from build123d import *

# Parameters (mm, degrees)
SKETCH1_R           = 1.7
BOSS_EXTRUDE1_DEPTH = 6.35
CHAMFER1_SIZE       = 1.7
SKETCH2_R           = 1.65
CUT_EXTRUDE1_DEPTH  = 10
FILLET1_R           = 3


with BuildPart() as part:
    # Sketch1 → Boss-Extrude1 (new body)
    with BuildSketch(Plane(origin=(7.6e-08, 0, -21.644897171), x_dir=(1, 0, 4e-09), z_dir=(-4e-09, 0, 1))):
        with BuildLine():
            Line((3.000021754, 7.262533291), (3.000021754, 1.9987))
            Line((3.000021754, 1.9987), (19.00000025, 1.9987))
            Line((19.00000025, 1.9987), (19.00000025, 22.8687))
            Line((19.00000025, 22.8687), (-19.00000025, 22.8687))
            Line((-19.00000025, 22.8687), (-19.00000025, 1.9987))
            Line((-19.00000025, 1.9987), (-3.409734271, 1.9987))
            Line((-3.409734271, 1.9987), (-3.409734271, 7.262533291))
            ThreePointArc((-3.409734271, 7.262533291), (-0.204856259, 10.467411304), (3.000021754, 7.262533291))
        make_face()
        with Locations((9.295143741, 7.262533291)):
            Circle(SKETCH1_R, mode=Mode.SUBTRACT)
        with Locations((-9.704856259, 7.262533291)):
            Circle(SKETCH1_R, mode=Mode.SUBTRACT)
    extrude(amount=BOSS_EXTRUDE1_DEPTH)

    # Chamfer1
    chamfer1_edges = [part.edges().sort_by_distance(p)[0] for p in [
        (7.595143795, 7.262533291, -15.294897144),
        (-11.404856205, 7.262533291, -15.294897211),
    ]]
    chamfer(chamfer1_edges, length=CHAMFER1_SIZE)

    # Sketch2 → Cut-Extrude1 (cut)
    with BuildSketch(Plane(origin=(0, 22.8687, 0), x_dir=(1, 0, 0), z_dir=(0, 1, 0))):
        with Locations((10, 18.469897104)):
            Circle(SKETCH2_R)
        with Locations((-10.042850258, 18.469897104)):
            Circle(SKETCH2_R)
    extrude(amount=-CUT_EXTRUDE1_DEPTH, mode=Mode.SUBTRACT)

    # Fillet1
    fillet1_edges = [part.edges().sort_by_distance(p)[0] for p in [
        (-3.409734206, 1.9987, -18.469897183),
        (-19.000000186, 1.9987, -18.469897237),
        (19.000000315, 1.9987, -18.469897104),
        (3.000021818, 1.9987, -18.46989716),
    ]]
    fillet(fillet1_edges, radius=FILLET1_R)


solid = part.part
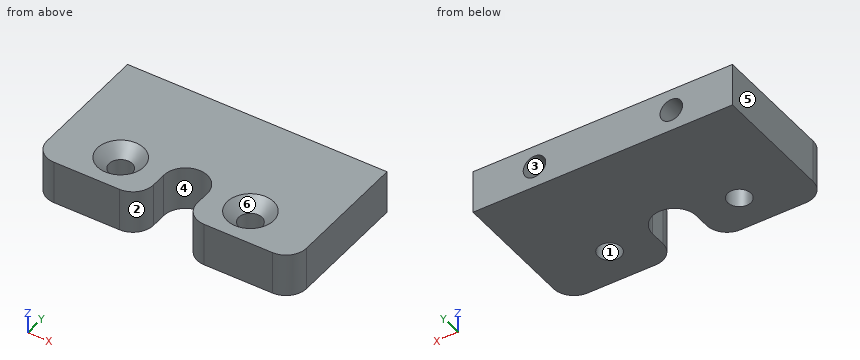
Could you check a few things on this model? Use its own coordinates, in mm. Face numbers are marked on the shaded views. A direction names the side the tool comes from. Coordinates: 2 decimals unless noted, no trailing zeros. Loops run counter-clockwise (first coordinate to the right, second up) from the corner with the lowest first, then second, coordinate; pieces in that order, holes last.
1. I need wall thicknesses on L1, parallel to X at y = 16, z = -18.5; L2, parallel to Z at x = 10, y = 16.75; L3, parallel to X at y = 13.75, z = -19.75. Which ranges of each line are inside material? Lowest first, please.
2. Imagine slicing it at A-A (z = -17.5). Please give me the cut outline in (x, y).
3. For P1, Ø2, axis at x = 10, z = -18.47, coming from the +Y side, with a flat end and sliding along its axis, tell me the tip position at first contact or that it passes through.
4. We'd pull the mould along Y, two halves only. Please class the marked faces 4, 5 and 6: released by +Y, released by -Y, zero draft, split by the parting line, or undercut.
5. For the marked faces 1, 2 and 3, which set-ups out of +Z, -Z, +X, -X, +Y, -Y let a thin tool reach every point of the face, with its end or its side?
6. Imagine slicing it at B-B (y = 21.5). Please give me the cut outline in (x, z), and give its area (3 significant figures).
7. Imagine slicing it at C-C (x = -5). Please give me the cut outline in (y, z).
Computed values:
1. L1: x = -19 to -11.69, -8.39 to 8.35, 11.65 to 19
1. L2: z = -21.64 to -20.12, -16.82 to -15.29
1. L3: x = -19 to -11.08, -9 to 8.96, 11.04 to 19
2. outline: (-19, 5) arc R3 ccw to (-16, 2) - (-6.41, 2) arc R3 ccw to (-3.41, 5) - (-3.41, 7.26) arc R3.2 cw to (3, 7.26) - (3, 5) arc R3 ccw to (6, 2) - (16, 2) arc R3 ccw to (19, 5) - (19, 22.87) - (11.33, 22.87) - (11.33, 12.87) - (8.67, 12.87) - (8.67, 22.87) - (-8.71, 22.87) - (-8.71, 12.87) - (-11.38, 12.87) - (-11.38, 22.87) - (-19, 22.87) - close; hole circle Ø3.4 at (-9.7, 7.26); hole circle Ø3.4 at (9.3, 7.26)
3. P1: stops at y = 12.87
4. face 4: released by -Y
4. face 5: zero draft
4. face 6: undercut
5. face 1: +Z, -Z
5. face 2: +Z, -Z, -Y
5. face 3: +Y
6. outline: (-19, -21.64) - (19, -21.64) - (19, -15.29) - (-19, -15.29) - close; hole circle Ø3.3 at (-10.04, -18.47); hole circle Ø3.3 at (10, -18.47)
6. area: 224 mm2
7. outline: (2.35, -21.64) - (22.87, -21.64) - (22.87, -15.29) - (2.35, -15.29) - close
